Source: CAD feature listing. Evaluate the final solid. Frame: model axes, mm. A direction names the side the tool comes from. Give positions to 0.01 mm unless a question says otherwise; leave off trailing zeros. Loops run counter-clockwise (first coordinate to the right, second up) from the corner with the lowest first, then second, coordinate; pieces in that order, holes last. Notation, with made-up numbers: (16, 75) - (75, 75) arc R16 ccw to (75, 97) - close; hole circle Ø9 at (-4.75, 26.25). An arc over 180 degrees is marked (long way). Put each result on its own line as item: value.
```python
from build123d import *

# Parameters (mm, degrees)
BOX001_W          = 10
BOX001_H          = 10
BOX001_DEPTH      = 8
CYLINDER_R        = 2.7
CYLINDER_DEPTH    = 10
CYLINDER001_R     = 3.5
CYLINDER001_DEPTH = 10
BOX_W             = 16
BOX_H             = 16
BOX_DEPTH         = 10


with BuildPart() as cube001:
    # Box001 → Box001 (new body)
    with BuildSketch(Plane(origin=(-5, -5, 0), x_dir=(1, 0, 0), z_dir=(0, 0, 1))):
        with Locations((5, 5)):
            Rectangle(BOX001_W, BOX001_H)
    extrude(amount=BOX001_DEPTH)


with BuildPart() as cylinder:
    # Cylinder → Cylinder (new body)
    with BuildSketch(Plane(origin=(1.7, 0, 10), x_dir=(1, 0, 0), z_dir=(0, 0, 1))):
        Circle(CYLINDER_R)
    extrude(amount=CYLINDER_DEPTH)


with BuildPart() as cut:
    # Cylinder001 → Cylinder001 (new body)
    with BuildSketch(Plane.XY.offset(10)):
        Circle(CYLINDER001_R)
    extrude(amount=CYLINDER001_DEPTH)

    # Cut: cut Cylinder
    add(cylinder.part, mode=Mode.SUBTRACT)


with BuildPart() as cut001:
    # Box → Box (new body)
    with BuildSketch(Plane(origin=(-8, -8, 0), x_dir=(1, 0, 0), z_dir=(0, 0, 1))):
        with Locations((8, 8)):
            Rectangle(BOX_W, BOX_H)
    extrude(amount=BOX_DEPTH)

    # Fusion: union Cut
    add(cut.part)

    # Cut001: cut Cube001
    add(cube001.part, mode=Mode.SUBTRACT)


solid = cut001.part
```
1) Section query A-A, the plane z = 6. Output: boundary loops of the cut face in (x, y), plus the area to 3 significant figures.
Check result:
outline: (-8, -8) - (8, -8) - (8, 8) - (-8, 8) - close; hole (-5, -5) - (5, -5) - (5, 5) - (-5, 5) - close
area: 156 mm²
2) Material intervals for line 1 along Y through (x, z) = (-3.25, 3); line 2 along Z through (x, y) = (4.25, -1), sorted ascending. Write a range as [from, to].
Check result:
line 1: [-8, -5], [5, 8]
line 2: [8, 10]
3) Mould query, pull axis X, two halves, no side actions, for faces 1 (the flat face through (-0.1, 5.4, 0)), 2 (the flat face through (0, 0, 8)), 3 (the flat face through (-8, 0, 5)), 4 (the flat face through (5, 0, 4)). Classes: pulls with the +X half, pulls with the -X half, needs draft (parallel to the pull), parting line crosses it, or undercut.
Check result:
face 1: needs draft
face 2: undercut
face 3: pulls with the -X half
face 4: undercut
4) Pin query (flat end, axial travel): P1, Ø3, axis at x = 0, y = -2, coming from the -Z side; P2, Ø1.5, axis at x = 1, y = -6, coming from the +Z side. Return the tip coordinate at first contact, or that it passes through.
Check result:
P1: z = 8
P2: z = 10
5) Section query B-B, the plane y = 0. Output: boundary loops of the cut face in (x, z).
Check result:
outline: (-8, 0) - (-5, 0) - (-5, 8) - (5, 8) - (5, 0) - (8, 0) - (8, 10) - (-1, 10) - (-1, 20) - (-3.5, 20) - (-3.5, 10) - (-8, 10) - close
6) Section query C-C, the plane x = 3.5. Output: boundary loops of the cut face in (y, z), plus the area to 3 significant figures.
Check result:
outline: (-8, 0) - (-5, 0) - (-5, 8) - (5, 8) - (5, 0) - (8, 0) - (8, 10) - (-8, 10) - close
area: 80.0 mm²
7) Section query D-D, the plane y = -3.25. Output: boundary loops of the cut face in (x, z), plus the area to 3 significant figures.
Check result:
outline: (-8, 0) - (-5, 0) - (-5, 8) - (5, 8) - (5, 0) - (8, 0) - (8, 10) - (1.3, 10) - (1.3, 20) - (-1.3, 20) - (-1.3, 10) - (-8, 10) - close
area: 106 mm²
8) Access query for faces 5 (the flat face through (0, 5, 4)), 6 (the cylindrical face through (-1, 0, 15)), 7 (the flat face through (0, 8, 5)). Directions: +Z, -Z, +X, -X, +Y, -Y. A direction counts if a zero-diameter tool reaches every point of the face in a straight line with its end or side. Return the directions, or none.
Check result:
face 5: -Z
face 6: +Z
face 7: +Z, -Z, +X, -X, +Y
